For this review, use the dimensioned drawing (mm, ordinates from the lowest corner) and the shaded views. Give positions to 0.01 mm unless a question says otherwise; leave off trailing zeros. Write each loop counter-clockwise with the first axis right and the second up, starting at its lowest first coordinate (ties: lowest second). Pieces come first, ordered by that corner, then holes. Notation, with made-up numbers: (42.5, 48.25) -> (101.5, 48.25) arc R31 cw to (101.5, 78.25) -> close; hole circle Ø11 at (30, -13). An arc over 180 degrees is marked (long way). Answer as CSV lines item,"result".
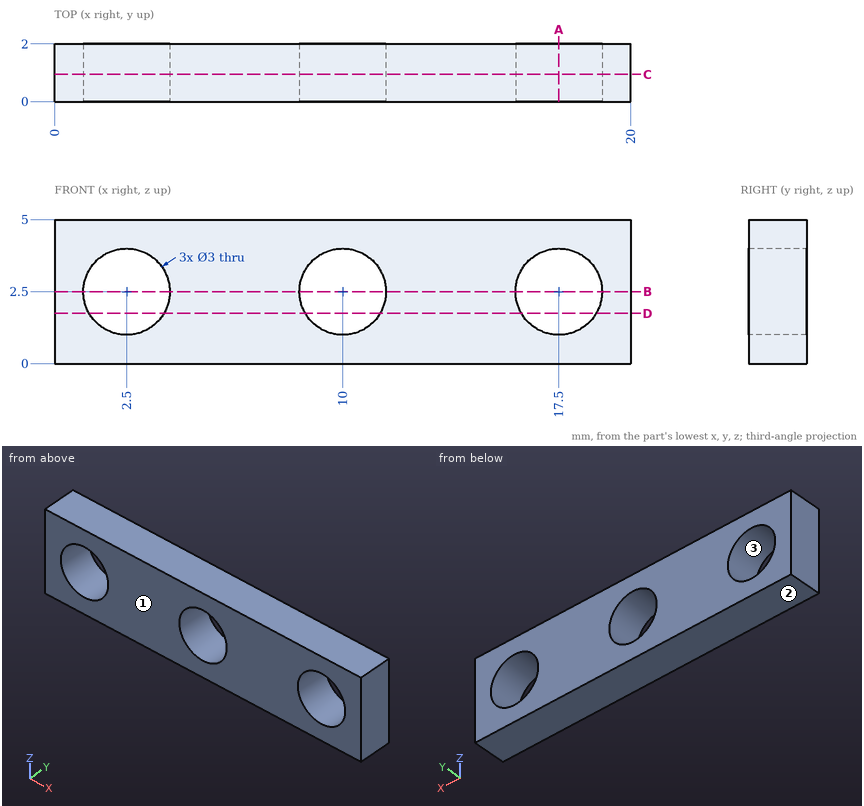
Q1. Add section A-A (x = 17.5). Write out the cut boundary in (y, z), plus the area to 3 significant figures.
Answer block:
outline,"(0, 0) -> (2, 0) -> (2, 1) -> (0, 1) -> close; (0, 4) -> (2, 4) -> (2, 5) -> (0, 5) -> close"
area,"4.00 mm2"
Q2. Add section D-D (z = 1.75). Write out the cut boundary in (x, y).
Answer block:
outline,"(0, 0) -> (1.2, 0) -> (1.2, 2) -> (0, 2) -> close; (3.8, 0) -> (8.7, 0) -> (8.7, 2) -> (3.8, 2) -> close; (11.3, 0) -> (16.2, 0) -> (16.2, 2) -> (11.3, 2) -> close; (18.8, 0) -> (20, 0) -> (20, 2) -> (18.8, 2) -> close"
Q3. Add section C-C (y = 0.95). Write out the cut boundary in (x, z), plus the area to 3 significant figures.
Answer block:
outline,"(0, 0) -> (20, 0) -> (20, 5) -> (0, 5) -> close; hole circle Ø3 at (2.5, 2.5); hole circle Ø3 at (10, 2.5); hole circle Ø3 at (17.5, 2.5)"
area,"78.8 mm2"
Q4. To check wall thickness, follow probe 1 along X at (y, z) = (1.2, 2.5); probe 2 along X at (y, z) = (1.3, 2); probe 3 along Z at (x, y) = (18.25, 1.2). State the ranges of each line that lie inside material, in increasing order. Write a range as [from, to].
Answer block:
probe 1,"x = [0, 1], [4, 8.5], [11.5, 16], [19, 20]"
probe 2,"x = [0, 1.09], [3.91, 8.59], [11.41, 16.09], [18.91, 20]"
probe 3,"z = [0, 1.2], [3.8, 5]"
Q5. Add section B-B (z = 2.5). Write out the cut boundary in (x, y), plus the area to 3 significant figures.
Answer block:
outline,"(0, 0) -> (1, 0) -> (1, 2) -> (0, 2) -> close; (4, 0) -> (8.5, 0) -> (8.5, 2) -> (4, 2) -> close; (11.5, 0) -> (16, 0) -> (16, 2) -> (11.5, 2) -> close; (19, 0) -> (20, 0) -> (20, 2) -> (19, 2) -> close"
area,"22.0 mm2"
Q6. Draft analysis for pull direction Z (two halves, no side actions). For the marked faces 1, 2 and 3, state which applies: released by +Z, released by -Z, zero draft, split by the parting line, or undercut.
Answer block:
face 1,"zero draft"
face 2,"released by -Z"
face 3,"undercut"
